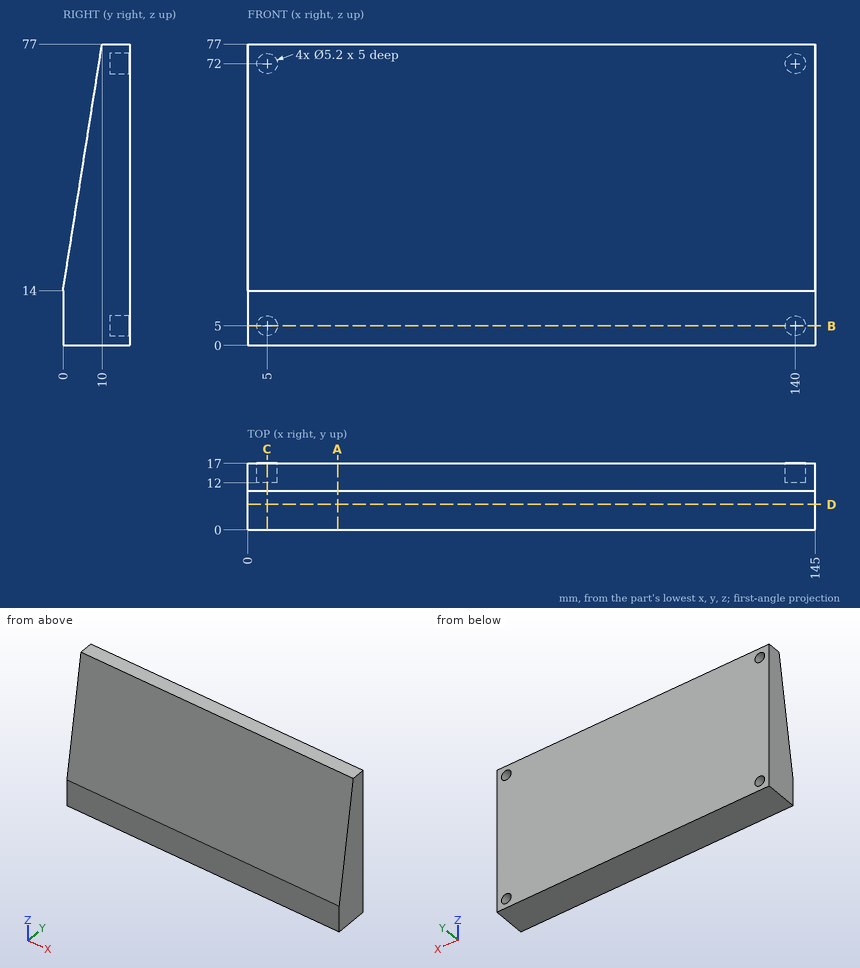
Job drawing, mm, ordinate dimensions from the low corner. One solid piece. Give positions to 0.01 mm unless a question says otherwise; leave off trailing zeros. Loops run counter-clockwise (first coordinate to the right, second up) from the corner with the lowest first, then second, coordinate; pieces in that order, holes last. Notation, with made-up numbers: M 84.5,-4 L 129.5,-4 A21 cw 129.5,17 Z; hole C 0,6 d10. An arc over 180 degrees is marked long. Answer in a Markdown table with one row per item. Add a question column.
Item 1: Band-saw the part on D-D on y = 6.5. Give the cut face in (x, z).
Item 2: Band-saw the part on C-C on x = 5. Give the cut face in (y, z), then the cut area to 3 significant figures.
Item 3: Drop flat-ended pins along their axis: P1, Ø1.6, axis at x = 141, z = 72.5, coming from the +Y side; P2, Ø4, axis at x = 36.5, z = 56, coming from the -Y side. Give the stop position or say it passes through.
Item 4: Band-saw the part on A-A on x = 23. Give the cut face in (y, z), then the cut area to 3 significant figures.
Item 5: Band-saw the part on B-B on z = 5. Give the cut face in (x, y).
Item 6: Probe probe 1 along X at (y, z) = (14.9, 5); probe 2 along Y at (x, z) = (84, 52.5); probe 3 along Y at (x, z) = (63.5, 35.5). List the from-to ranges inside material, lowest first.
Reply:
| question | item | result |
|---|---|---|
| 1 | outline | M 0,0 L 145,0 L 145,54.95 L 0,54.95 Z |
| 2 | outline | M 0,0 L 17,0 L 17,2.4 L 12,2.4 L 12,7.6 L 17,7.6 L 17,69.4 L 12,69.4 L 12,74.6 L 17,74.6 L 17,77 L 10,77 L 0,14 Z |
| 2 | area | 942 mm^2 |
| 3 | P1 | stops at y = 12 |
| 3 | P2 | stops at y = 6.35 |
| 4 | outline | M 0,0 L 17,0 L 17,77 L 10,77 L 0,14 Z |
| 4 | area | 994 mm^2 |
| 5 | outline | M 0,0 L 145,0 L 145,17 L 142.6,17 L 142.6,12 L 137.4,12 L 137.4,17 L 7.6,17 L 7.6,12 L 2.4,12 L 2.4,17 L 0,17 Z |
| 6 | probe 1 | x = 0 to 2.4, 7.6 to 137.4, 142.6 to 145 |
| 6 | probe 2 | y = 6.11 to 17 |
| 6 | probe 3 | y = 3.41 to 17 |
